from build123d import *

# Parameters (mm, degrees)
F0_R     = 8
F1_DEPTH = 6
F2_R     = 8
F2_R_2   = 6
F3_DEPTH = 0.5
F4_R     = 1


with BuildPart() as f1:
    # F0 (on Top) → F1 (new body)
    with BuildSketch(Plane.XY):
        with BuildLine():
            Line((8.660254, -30), (30.310889, 7.5))
            ThreePointArc((30.310889, 7.5), (30.310889, 17.5), (21.650635, 22.5))
            Line((21.650635, 22.5), (-21.650635, 22.5))
            ThreePointArc((-21.650635, 22.5), (-30.310889, 17.5), (-30.310889, 7.5))
            Line((-30.310889, 7.5), (-8.660254, -30))
            ThreePointArc((-8.660254, -30), (0, -35), (8.660254, -30))
        make_face()
        Polygon((-3.406367, -16.6), (3.406367, -16.6), (6.812733, -22.5), (3.406367, -28.4), (-3.406367, -28.4), (-6.812733, -22.5), align=None, mode=Mode.SUBTRACT)
        Circle(F0_R, mode=Mode.SUBTRACT)
        Polygon((-16.079205, 17.15), (-12.672838, 11.25), (-16.079205, 5.35), (-22.891938, 5.35), (-26.298305, 11.25), (-22.891938, 17.15), align=None, mode=Mode.SUBTRACT)
        Polygon((22.891938, 5.35), (16.079205, 5.35), (12.672838, 11.25), (16.079205, 17.15), (22.891938, 17.15), (26.298305, 11.25), align=None, mode=Mode.SUBTRACT)
    extrude(amount=F1_DEPTH)

    # F2 (on Top) → F3 (join)
    with BuildSketch(Plane.XY):
        Circle(F2_R)
        Circle(F2_R_2, mode=Mode.SUBTRACT)
    extrude(amount=F3_DEPTH)

    # F4
    f4_edges = [f1.edges().sort_by_distance(p)[0] for p in [
        (0, 22.5, 6),
        (0, 22.5, 0),
    ]]
    fillet(f4_edges, radius=F4_R)


solid = f1.part
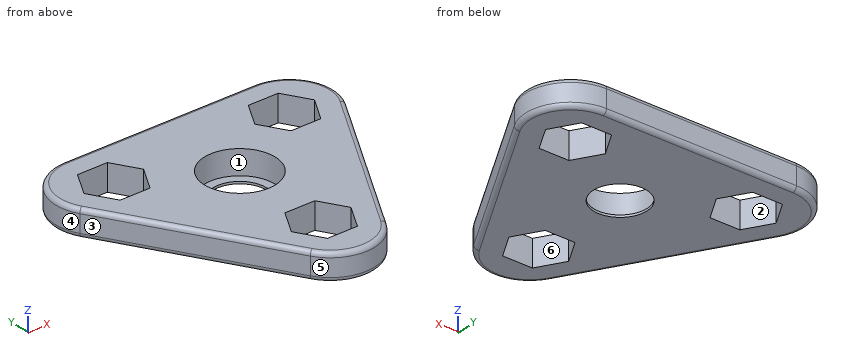
Build history of the part. All positions in model axes, mm. Face numbers are marked on the shaded views. A direction names the side the tool comes from. Give positions to 0.01 mm unless a question says otherwise; leave off trailing zeros. Loops run counter-clockwise (first coordinate to the right, second up) from the corner with the lowest first, then second, coordinate; pieces in that order, holes last. Notation, with made-up numbers: (-20, -30) - (-3, -30) arc R17 ccw to (-3, -17) - close; hole circle Ø2 at (55.25, -6.75). An arc over 180 degrees is marked (long way). Write item = value, one per line. Start each with the question number.
1) Tool access for the marked faces 1, 2 and 3: list every direction of +Z, -Z, +X, -X, +Y, -Y with a clear straight run to the whole face (end or side of a thin tool).
2) Pull direction X, two halves, no side cores. Call the marked faces 4, 5 and 6: +X half, -X half, draft (parallel to the pull), parting line (faces both ways), or undercut.
3) Band-saw the part on A-A on z = 3.65. Give the cut face in (x, y).
4) Probe probe 1 along Y at (x, z) = (0, 3.4); probe 2 along Y at (x, z) = (2, 3.65); probe 3 along X at (y, z) = (17, 0.45). List the from-to ranges inside material, lowest first. Write a range as from..to.
5) Band-saw the part on C-C on y = 10.5. Count the separate pieces of the cut face and the enclosed holes in it, plus the area to 3 significant figures.
6) Band-saw the part on B-B on x = 0. Give the cut face in (y, z), plus the area to 3 significant figures.
7) Drop a flat-ended pin along its axis: pin 1 Ø3 at (x, z) = (21, 3) entering from -Y (3 decimals). Give the stop position or say it passes through.
Final values:
q1.face_1 = +Z
q1.face_2 = +Z, -Z
q1.face_3 = +Z, -Z, -X, -Y
q2.face_4 = -X half
q2.face_5 = parting line
q2.face_6 = undercut
q3.outline = (-30.31, 7.5) - (-8.66, -30) arc R10 ccw to (8.66, -30) - (30.31, 7.5) arc R10 ccw to (21.65, 22.5) - (-21.65, 22.5) arc R10 ccw to start; hole (-26.3, 11.25) - (-22.89, 5.35) - (-16.08, 5.35) - (-12.67, 11.25) - (-16.08, 17.15) - (-22.89, 17.15) - close; hole circle Ø16 at (0, 0); hole (-6.81, -22.5) - (-3.41, -28.4) - (3.41, -28.4) - (6.81, -22.5) - (3.41, -16.6) - (-3.41, -16.6) - close; hole (12.67, 11.25) - (16.08, 5.35) - (22.89, 5.35) - (26.3, 11.25) - (22.89, 17.15) - (16.08, 17.15) - close
q4.probe_1 = -35..-28.4, -16.6..-8, 8..22.5
q4.probe_2 = -34.8..-28.4, -16.6..-7.75, 7.75..22.5
q4.probe_3 = -30.4..-22.98, -15.99..15.99, 22.98..30.4
q5.separate_pieces = 3
q5.enclosed_holes = 0
q5.area = 223 mm²
q6.outline = (-35, 1) arc R1 ccw to (-34, 0) - (-28.4, 0) - (-28.4, 6) - (-34, 6) arc R1 ccw to (-35, 5) - close; (-16.6, 0) - (-6, 0) - (-6, 0.5) - (-8, 0.5) - (-8, 6) - (-16.6, 6) - close; (6, 0) - (21.5, 0) arc R1 ccw to (22.5, 1) - (22.5, 5) arc R1 ccw to (21.5, 6) - (8, 6) - (8, 0.5) - (6, 0.5) - close
q6.area = 179 mm²
q7.pin_1 = -11.225
